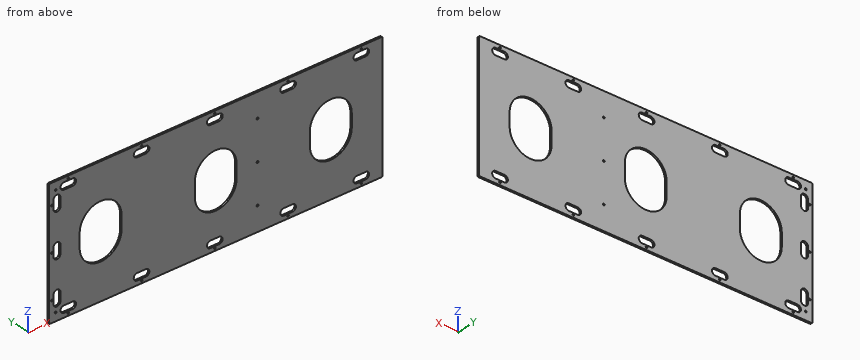
```python
from build123d import *

# Parameters (mm, degrees)
SKETCH1_W           = 1212.85
SKETCH1_H           = 469.9
BOSS_EXTRUDE1_DEPTH = 6.35
CUT_EXTRUDE1_DEPTH  = 1301.711903152
SKETCH4_R           = 3.175
CUT_EXTRUDE3_DEPTH  = 1301.711903152
LPATTERN1_OUTLINE_R = 3.175
LPATTERN1_DEPTH     = 6.35
FILLET1_R           = 2.54
SKETCH5_R           = 3.3782
CUT_EXTRUDE4_DEPTH  = 6.35


# Read off the part's stored shape, not the designer's step: LPattern1
with BuildPart() as part:
    # Sketch1 → Boss-Extrude1 (new body)
    with BuildSketch(Plane(origin=(0, 0, 0), x_dir=(1, 0, 0), z_dir=(0, 1, 0))):
        with Locations((606.425, 234.95)):
            Rectangle(SKETCH1_W, SKETCH1_H)
    extrude(amount=BOSS_EXTRUDE1_DEPTH)

    # Sketch2 → Cut-Extrude1 (cut, through all)
    with BuildSketch(Plane(origin=(0, 6.35, 0), x_dir=(1, 0, 0), z_dir=(0, 1, 0))):
        with BuildLine():
            Line((263.525, 260.35), (263.525, 209.55))
            ThreePointArc((263.525, 209.55), (187.325, 133.35), (111.125, 209.55))
            Line((111.125, 209.55), (111.125, 260.35))
            ThreePointArc((111.125, 260.35), (187.325, 336.55), (263.525, 260.35))
        make_face()
        with BuildLine():
            Line((682.625, 260.35), (682.625, 209.55))
            ThreePointArc((682.625, 209.55), (606.425, 133.35), (530.225, 209.55))
            Line((530.225, 209.55), (530.225, 260.35))
            ThreePointArc((530.225, 260.35), (606.425, 336.55), (682.625, 260.35))
        make_face()
        with BuildLine():
            Line((1101.725, 260.35), (1101.725, 209.55))
            ThreePointArc((1101.725, 209.55), (1025.525, 133.35), (949.325, 209.55))
            Line((949.325, 209.55), (949.325, 260.35))
            ThreePointArc((949.325, 260.35), (1025.525, 336.55), (1101.725, 260.35))
        make_face()
    extrude(amount=-CUT_EXTRUDE1_DEPTH, mode=Mode.SUBTRACT)

    # Sketch4 → Cut-Extrude3 (cut, through all)
    with BuildSketch(Plane(origin=(0, 6.35, 0), x_dir=(1, 0, 0), z_dir=(0, 1, 0))):
        with Locations(Location((9.525, 393.7, 0), (0, 0, 270))):
            Circle(SKETCH4_R)
        with Locations(Location((9.525, 234.95, 0), (0, 0, 270))):
            Circle(SKETCH4_R)
        with Locations(Location((9.525, 76.2, 0), (0, 0, 270))):
            Circle(SKETCH4_R)
        with Locations(Location((69.85, 460.375, 0), (0, 0, 270))):
            Circle(SKETCH4_R)
        with Locations(Location((69.85, 9.525, 0), (0, 0, 270))):
            Circle(SKETCH4_R)
        with BuildLine():
            Line((41.275, 250.825), (41.275, 219.075))
            ThreePointArc((41.275, 219.075), (28.575, 206.375), (15.875, 219.075))
            Line((15.875, 219.075), (15.875, 250.825))
            ThreePointArc((15.875, 250.825), (28.575, 263.525), (41.275, 250.825))
        make_face()
        with BuildLine():
            Line((53.975, 454.025), (85.725, 454.025))
            ThreePointArc((85.725, 454.025), (98.425, 441.325), (85.725, 428.625))
            Line((85.725, 428.625), (53.975, 428.625))
            ThreePointArc((53.975, 428.625), (41.275, 441.325), (53.975, 454.025))
        make_face()
        with BuildLine():
            Line((53.975, 41.275), (85.725, 41.275))
            ThreePointArc((85.725, 41.275), (98.425, 28.575), (85.725, 15.875))
            Line((85.725, 15.875), (53.975, 15.875))
            ThreePointArc((53.975, 15.875), (41.275, 28.575), (53.975, 41.275))
        make_face()
        with BuildLine():
            Line((15.875, 60.325), (15.875, 92.075))
            ThreePointArc((15.875, 92.075), (28.575, 104.775), (41.275, 92.075))
            Line((41.275, 92.075), (41.275, 60.325))
            ThreePointArc((41.275, 60.325), (28.575, 47.625), (15.875, 60.325))
        make_face()
        with BuildLine():
            Line((15.875, 377.825), (15.875, 409.575))
            ThreePointArc((15.875, 409.575), (28.575, 422.275), (41.275, 409.575))
            Line((41.275, 409.575), (41.275, 377.825))
            ThreePointArc((41.275, 377.825), (28.575, 365.125), (15.875, 377.825))
        make_face()
    extrude(amount=-CUT_EXTRUDE3_DEPTH, mode=Mode.SUBTRACT)

    # LPattern1 outline → LPattern1 (cut)
    with BuildSketch(Plane(origin=(0, 0, 0), x_dir=(1, 0, 0), z_dir=(0, 1, 0))):
        with BuildLine():
            ThreePointArc((1120.775, 454.025), (1108.075, 441.325), (1120.775, 428.625))
            Line((1120.775, 428.625), (1152.525, 428.625))
            ThreePointArc((1152.525, 428.625), (1165.225, 441.325), (1152.525, 454.025))
            Line((1152.525, 454.025), (1120.775, 454.025))
        make_face()
        with BuildLine():
            ThreePointArc((854.075, 454.025), (841.375, 441.325), (854.075, 428.625))
            Line((854.075, 428.625), (885.825, 428.625))
            ThreePointArc((885.825, 428.625), (898.525, 441.325), (885.825, 454.025))
            Line((885.825, 454.025), (854.075, 454.025))
        make_face()
        with BuildLine():
            ThreePointArc((587.375, 454.025), (574.675, 441.325), (587.375, 428.625))
            Line((587.375, 428.625), (619.125, 428.625))
            ThreePointArc((619.125, 428.625), (631.825, 441.325), (619.125, 454.025))
            Line((619.125, 454.025), (587.375, 454.025))
        make_face()
        with BuildLine():
            ThreePointArc((320.675, 454.025), (307.975, 441.325), (320.675, 428.625))
            Line((320.675, 428.625), (352.425, 428.625))
            ThreePointArc((352.425, 428.625), (365.125, 441.325), (352.425, 454.025))
            Line((352.425, 454.025), (320.675, 454.025))
        make_face()
        with BuildLine():
            ThreePointArc((1120.775, 41.275), (1108.075, 28.575), (1120.775, 15.875))
            Line((1120.775, 15.875), (1152.525, 15.875))
            ThreePointArc((1152.525, 15.875), (1165.225, 28.575), (1152.525, 41.275))
            Line((1152.525, 41.275), (1120.775, 41.275))
        make_face()
        with BuildLine():
            ThreePointArc((854.075, 41.275), (841.375, 28.575), (854.075, 15.875))
            Line((854.075, 15.875), (885.825, 15.875))
            ThreePointArc((885.825, 15.875), (898.525, 28.575), (885.825, 41.275))
            Line((885.825, 41.275), (854.075, 41.275))
        make_face()
        with BuildLine():
            ThreePointArc((587.375, 41.275), (574.675, 28.575), (587.375, 15.875))
            Line((587.375, 15.875), (619.125, 15.875))
            ThreePointArc((619.125, 15.875), (631.825, 28.575), (619.125, 41.275))
            Line((619.125, 41.275), (587.375, 41.275))
        make_face()
        with BuildLine():
            ThreePointArc((320.675, 41.275), (307.975, 28.575), (320.675, 15.875))
            Line((320.675, 15.875), (352.425, 15.875))
            ThreePointArc((352.425, 15.875), (365.125, 28.575), (352.425, 41.275))
            Line((352.425, 41.275), (320.675, 41.275))
        make_face()
        with Locations((1136.65, 9.525)):
            Circle(LPATTERN1_OUTLINE_R)
        with Locations((1136.65, 460.375)):
            Circle(LPATTERN1_OUTLINE_R)
        with Locations((869.95, 9.525)):
            Circle(LPATTERN1_OUTLINE_R)
        with Locations((869.95, 460.375)):
            Circle(LPATTERN1_OUTLINE_R)
        with Locations((603.25, 9.525)):
            Circle(LPATTERN1_OUTLINE_R)
        with Locations((603.25, 460.375)):
            Circle(LPATTERN1_OUTLINE_R)
        with Locations((336.55, 9.525)):
            Circle(LPATTERN1_OUTLINE_R)
        with Locations((336.55, 460.375)):
            Circle(LPATTERN1_OUTLINE_R)
    extrude(amount=LPATTERN1_DEPTH, mode=Mode.SUBTRACT)

    # Fillet1
    fillet1_edges = [part.edges().sort_by_distance(p)[0] for p in [
        (0, 3.175, 0),
        (0, 3.175, -469.9),
        (1212.85, 3.175, -469.9),
        (1212.85, 3.175, 0),
    ]]
    fillet(fillet1_edges, radius=FILLET1_R)

    # Sketch5 → Cut-Extrude4 (cut)
    with BuildSketch(Plane(origin=(0, 6.35, 0), x_dir=(1, 0, 0), z_dir=(0, 1, 0))):
        with Locations(Location((23.8125, 439.7375, 0), (0, 0, 270))):
            Circle(SKETCH5_R)
        with Locations(Location((23.8125, 30.1625, 0), (0, 0, 270))):
            Circle(SKETCH5_R)
        with Locations(Location((758.825, 89.154, 0), (0, 0, 270))):
            Circle(SKETCH5_R)
        with Locations(Location((758.825, 234.95, 0), (0, 0, 270))):
            Circle(SKETCH5_R)
        with Locations(Location((758.825, 380.746, 0), (0, 0, 270))):
            Circle(SKETCH5_R)
    extrude(amount=-CUT_EXTRUDE4_DEPTH, mode=Mode.SUBTRACT)


solid = part.part
```
Input: part model. Units: mm. Frame: model coordinates. Coordinates: 2 decimals unless noted, no trailing zeros. Loops run counter-clockwise (first coordinate to the right, second up) from the corner with the lowest first, then second, coordinate; pieces in that order, holes last. Notation, with made-up numbers: M -39.5,46 L -12.5,46 A16 cw -12.5,58 Z; hole C 50,39 d6. An arc over 180 degrees is marked long. Use a Markdown table: item, result. Add a question column.
1) Line query: L1, parallel to X at y = 4.5, z = -225.5 (3 decimals); L2, parallel to X at y = 1.75, z = -76.2 (3 decimals); L3, parallel to Z at x = 1136.65, y = 5 (3 decimals). Output: solid intervals per line, ascending. Write a range as from..to.
2) Section C-C, the plane y = 2.75. Give the number of separate pieces and of enclosed holes in the cut face, plus the area to 3 significant figures.
3) Section A-A, the plane x = 651.5. Return the cut outline in (y, z), plus the area to 3 significant figures.
4) Section B-B, the plane x = 149.5. Return the cut outline in (y, z).
Answer below:
| question | item | result |
|---|---|---|
| 1 | L1 | 0..15.875, 41.275..111.125, 263.525..530.225, 682.625..949.325, 1101.725..1212.85 |
| 1 | L2 | 0..6.35, 12.7..15.875, 41.275..1212.85 |
| 1 | L3 | -469.9..-463.55, -457.2..-454.025, -428.625..-41.275, -15.875..-12.7, -6.35..0 |
| 2 | separate pieces | 1 |
| 2 | enclosed holes | 34 |
| 2 | area | 474,000 mm2 |
| 3 | outline | M 0,-469.9 L 6.35,-469.9 L 6.35,-321.79 L 0,-321.79 Z; M 0,-148.11 L 6.35,-148.11 L 6.35,0 L 0,0 Z |
| 3 | area | 1,880 mm2 |
| 4 | outline | M 0,-469.9 L 6.35,-469.9 L 6.35,-326.5 L 0,-326.5 Z; M 0,-143.4 L 6.35,-143.4 L 6.35,0 L 0,0 Z |
